Can you work these out from the model? Positions are in its coordinate system, mm. Face numbers are marked on the shaded views. A direction names the side the tool comes from. Coordinates: 2 decimals unless noted, no trailing zeros. Order: outer loops, then holes, each group sorted by start corner. A loop starts at its lowest first (then second) coordinate and runs counter-clockwise, first axis right, second up. Notation, with made-up numbers: (55.5, 87) -> (59.5, 87) arc R7 cw to (59.5, 91) -> close; hole circle Ø10 at (36.25, 29). An arc over 180 degrees is marked (long way). Answer in a Markdown table with one row per item.
```python
from build123d import *

# Parameters (mm, degrees)
SKETCH006_R     = 41.5
SKETCH006_R_2   = 1.5
SKETCH006_R_3   = 4
PAD_DEPTH       = 4
SKETCH007_R     = 38.5
SKETCH007_R_2   = 1.5
SKETCH007_R_3   = 4
PAD001_DEPTH    = 1
SKETCH008_R     = 43
SKETCH008_R_2   = 1.5
SKETCH008_R_3   = 4
PAD002_DEPTH    = 1
SKETCH_R        = 31
SKETCH_R_2      = 10
POCKET_DEPTH    = 4
CHAMFER_SIZE    = 0.9
CHAMFER001_SIZE = 3
CHAMFER002_SIZE = 2


with BuildPart() as part:
    # Sketch006 → Pad (new body)
    with BuildSketch(Plane.XY.offset(22)):
        Circle(SKETCH006_R)
        with Locations((0, 36)):
            Circle(SKETCH006_R_2, mode=Mode.SUBTRACT)
        with Locations((31.176915, -18)):
            Circle(SKETCH006_R_2, mode=Mode.SUBTRACT)
        with Locations((-31.176915, -18)):
            Circle(SKETCH006_R_2, mode=Mode.SUBTRACT)
        Circle(SKETCH006_R_3, mode=Mode.SUBTRACT)
    extrude(amount=PAD_DEPTH)

    # Sketch007 → Pad001 (join)
    with BuildSketch(Plane.XY.offset(22)):
        Circle(SKETCH007_R)
        with Locations((0, 36)):
            Circle(SKETCH007_R_2, mode=Mode.SUBTRACT)
        with Locations((31.176915, -18)):
            Circle(SKETCH007_R_2, mode=Mode.SUBTRACT)
        with Locations((-31.176915, -18)):
            Circle(SKETCH007_R_2, mode=Mode.SUBTRACT)
        Circle(SKETCH007_R_3, mode=Mode.SUBTRACT)
    extrude(amount=-PAD001_DEPTH)

    # Sketch008 → Pad002 (join)
    with BuildSketch(Plane.XY.offset(26)):
        Circle(SKETCH008_R)
        with Locations((0, 36)):
            Circle(SKETCH008_R_2, mode=Mode.SUBTRACT)
        with Locations((31.176915, -18)):
            Circle(SKETCH008_R_2, mode=Mode.SUBTRACT)
        with Locations((-31.176915, -18)):
            Circle(SKETCH008_R_2, mode=Mode.SUBTRACT)
        Circle(SKETCH008_R_3, mode=Mode.SUBTRACT)
    extrude(amount=PAD002_DEPTH)

    # Sketch (on Face6 of Pad002) → Pocket (cut)
    with BuildSketch(Plane(origin=(0, 0, 21), x_dir=(1, 0, 0), z_dir=(0, 0, -1))):
        Circle(SKETCH_R)
        Circle(SKETCH_R_2, mode=Mode.SUBTRACT)
    extrude(amount=-POCKET_DEPTH, mode=Mode.SUBTRACT)

    # Chamfer
    chamfer_edges = [part.edges().sort_by_distance(p)[0] for p in [
        (-4, 0, 21),
    ]]
    chamfer(chamfer_edges, length=CHAMFER_SIZE)

    # Chamfer001
    chamfer001_edges = [part.edges().sort_by_distance(p)[0] for p in [
        (-10, 0, 25),
    ]]
    chamfer(chamfer001_edges, length=CHAMFER001_SIZE)

    # Chamfer002
    chamfer002_edges = [part.edges().sort_by_distance(p)[0] for p in [
        (-31, 0, 25),
    ]]
    chamfer(chamfer002_edges, length=CHAMFER002_SIZE)


solid = part.part
```
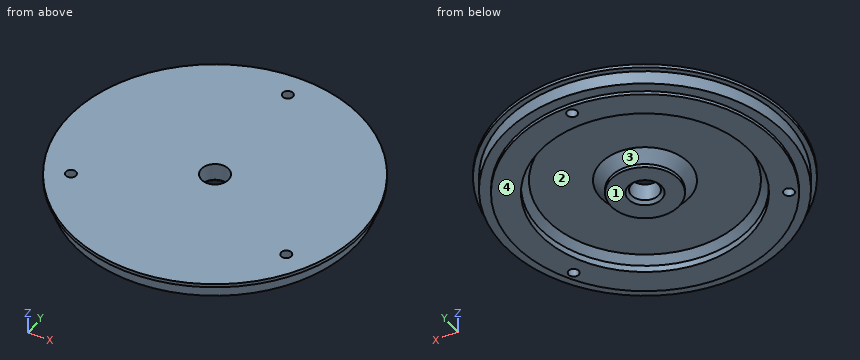
(1) On a 3-axis mill with a long thin cutter (end or side, diameter ignored), from which of +Z, -Z, +X, -X, +Y, -Y can I reach the whole of each face in a straight line? I mean the marked faces 1 and 2. Say none if no direction works.
Response values:
| item | result |
|---|---|
| face 1 | -Z, +X, -X, +Y, -Y |
| face 2 | -Z |
(2) Suppose I cut it at C-C (x = 0). Count the separate pieces of the cut face and the enclosed holes in it, and give its area (3 significant figures).
Response values:
| item | result |
|---|---|
| separate pieces | 3 |
| enclosed holes | 0 |
| area | 273 mm2 |
(3) I need wall thicknesses on line 1 (Y direction, x = 0, z = 25.6); line 2 (Y direction, x = 0, z = 23.65); line 3 (X direction, y = -4.5, z = 21.6). Which ranges of each line are inside material? Lowest first, please. Write a range as [from, to].
Response values:
| item | result |
|---|---|
| line 1 | [-41.5, -4], [4, 34.5], [37.5, 41.5] |
| line 2 | [-41.5, -30.35], [-11.65, -4], [4, 11.65], [30.35, 34.5], [37.5, 41.5] |
| line 3 | [-38.24, -30.67], [-8.93, 8.93], [30.67, 38.24] |
(4) Suppose I cut it at A-A (z = 23.95). Please give me the cut outline in (x, y), and give its area (3 significant figures).
Response values:
| item | result |
|---|---|
| outline | circle Ø83 at (0, 0); circle Ø23.9 at (0, 0); hole circle Ø3 at (-31.18, -18); hole circle Ø60.1 at (0, 0); hole circle Ø8 at (0, 0); hole circle Ø3 at (0, 36); hole circle Ø3 at (31.18, -18) |
| area | 2,950 mm2 |
(5) Suppose I cut it at D-D (y = -36). Please give me the cut outline in (x, z).
Response values:
| item | result |
|---|---|
| outline | (-23.52, 26) -> (-20.65, 26) -> (-20.65, 22) -> (-13.65, 22) -> (-13.65, 21) -> (13.65, 21) -> (13.65, 22) -> (20.65, 22) -> (20.65, 26) -> (23.52, 26) -> (23.52, 27) -> (-23.52, 27) -> close |
(6) We'd pull the mould along X, two halves only. Please class the marked faces 3 and 4: +X half, -X half, draft (parallel to the pull), parting line (faces both ways), or undercut.
Response values:
| item | result |
|---|---|
| face 3 | undercut |
| face 4 | draft |
(7) Will these pins go through, and if not, where does the flat tip stop? pin 1 Ø3 at (y, z) = (-27.5, 26) entering from -X; pin 2 Ø1 at (x, z) = (-17, 25) entering from +Y; pin 3 Ø3 at (x, y) = (-17.5, 21.5) entering from -Z.
Response values:
| item | result |
|---|---|
| pin 1 | x = -34.25 |
| pin 2 | y = 38.08 |
| pin 3 | z = 24.78 |
